from build123d import *

# Parameters (mm, degrees)
CROQUIS1_R              = 7.5
CROQUIS1_R_2            = 4.1
SALIENTE_EXTRUIR1_DEPTH = 24
CROQUIS2_W              = 0.35
CROQUIS2_H              = 1.1


with BuildPart() as part:
    # Croquis1 → Saliente-Extruir1 (new body)
    with BuildSketch(Plane(origin=(0, 0, 0), x_dir=(1, 0, 0), z_dir=(0, 1, 0))):
        with Locations(Location((0, 0, 0), (0, 0, 270))):
            Circle(CROQUIS1_R)
        with Locations(Location((0, 0, 0), (0, 0, 270))):
            Circle(CROQUIS1_R_2, mode=Mode.SUBTRACT)
    extrude(amount=SALIENTE_EXTRUIR1_DEPTH)

    # Croquis2 → Cortar-Revolución1 (revolve, cut)
    with BuildSketch(Plane.XY, mode=Mode.PRIVATE) as cortar_revoluci_n1_sk:
        with Locations((-7.325, 20.15)):
            Rectangle(CROQUIS2_W, CROQUIS2_H)
        with Locations((-7.325, 3.85)):
            Rectangle(CROQUIS2_W, CROQUIS2_H)
    revolve(cortar_revoluci_n1_sk.sketch.rotate(Axis((0, 0, 0), (0, 1, 0)), 270), axis=Axis((0, 0, 0), (0, 1, 0)), mode=Mode.SUBTRACT)


solid = part.part
Input: part model. Units: mm. Frame: model coordinates. A direction names the side the tool comes from. Round coordinates to 2 decimals unless told otherwise and drop trailing zeros. Loops run counter-clockwise (first coordinate to the right, second up) from the corner with the lowest first, then second, coordinate; pieces in that order, holes last. Notation, with made-up numbers: (-12, 39.25) -> (10, 39.25) arc R7 cw to (10, 50.25) -> close; hole circle Ø7 at (-27.75, -14.75). An arc over 180 degrees is marked (long way). Answer as a JSON object with one key per item and string values. Group by question number.
1) Draft query along Y for faces 1 (the flat face through (-3.2, 24, 3.2)), 2 (the cylindrical face through (-7.09, 20.16, 0.93)), 3 (the flat face through (-3.2, 0, 3.2)), 4 (the cylindrical face through (4.065, 11.832, -0.534)). Return one class per face: +Y half, -Y half, draft (parallel to the pull), parting line (faces both ways), or undercut.
2) Section query C-C on y = 16.75. Output: boundary loops of the cut face in (x, z).
3) Section query B-B on x = 0. Output: boundary loops of the cut face in (y, z), plus the area to 3 significant figures.
4) Section query D-D on x = -5.25. Output: boundary loops of the cut face in (y, z).
5) Reachability of faces 5 (the cylindrical face through (0.33, 22.327, -7.493)), 6 (the cylindrical face through (-7.09, 3.86, 0.93)) from +Z, -Z, +X, -X, +Y, -Y: full face, straight path, thin tool, end or side. Return the list, or none.
6) Ray query, L1, parallel to X at y = 9.25, z = 0; L2, parallel to Z at x = 2.5, y = 7; L3, parallel to Z at x = -3.5, y = 6. Return the intervals inside material, ascending.
7) Section query A-A on z = 0. Output: boundary loops of the cut face in (x, y).
8) Pin query (flat end, axial travel): pin 1 (6 mm diameter, centred on y = 5.5, z = 5.5, fed in from -X); pin 2 (1.5 mm diameter, centred on x = 2, y = 9.5, fed in from -Z); pin 3 (1 mm diameter, centred on y = 7.5, z = -4.5, fed in from +X). Return the tip coordinate at first contact, or that it passes through.
Reply:
{
 "1": {"face 1": "+Y half", "face 2": "undercut", "face 3": "-Y half", "face 4": "draft"},
 "2": {"outline": "circle Ø15 at (0, 0); hole circle Ø8.2 at (0, 0)"},
 "3": {"outline": "(0, -7.5) -> (3.3, -7.5) -> (3.3, -7.15) -> (4.4, -7.15) -> (4.4, -7.5) -> (19.6, -7.5) -> (19.6, -7.15) -> (20.7, -7.15) -> (20.7, -7.5) -> (24, -7.5) -> (24, -4.1) -> (0, -4.1) -> close; (0, 4.1) -> (24, 4.1) -> (24, 7.5) -> (20.7, 7.5) -> (20.7, 7.15) -> (19.6, 7.15) -> (19.6, 7.5) -> (4.4, 7.5) -> (4.4, 7.15) -> (3.3, 7.15) -> (3.3, 7.5) -> (0, 7.5) -> close", "area": "162 mm2"},
 "4": {"outline": "(0, -5.36) -> (3.3, -5.36) -> (3.3, -4.85) -> (4.4, -4.85) -> (4.4, -5.36) -> (19.6, -5.36) -> (19.6, -4.85) -> (20.7, -4.85) -> (20.7, -5.36) -> (24, -5.36) -> (24, 5.36) -> (20.7, 5.36) -> (20.7, 4.85) -> (19.6, 4.85) -> (19.6, 5.36) -> (4.4, 5.36) -> (4.4, 4.85) -> (3.3, 4.85) -> (3.3, 5.36) -> (0, 5.36) -> close"},
 "5": {"face 5": "+Y, -Y", "face 6": "none"},
 "6": {"L1": "x = -7.5 to -4.1, 4.1 to 7.5", "L2": "z = -7.07 to -3.25, 3.25 to 7.07", "L3": "z = -6.63 to -2.14, 2.14 to 6.63"},
 "7": {"outline": "(-7.5, 0) -> (-4.1, 0) -> (-4.1, 24) -> (-7.5, 24) -> (-7.5, 20.7) -> (-7.15, 20.7) -> (-7.15, 19.6) -> (-7.5, 19.6) -> (-7.5, 4.4) -> (-7.15, 4.4) -> (-7.15, 3.3) -> (-7.5, 3.3) -> close; (4.1, 0) -> (7.5, 0) -> (7.5, 3.3) -> (7.15, 3.3) -> (7.15, 4.4) -> (7.5, 4.4) -> (7.5, 19.6) -> (7.15, 19.6) -> (7.15, 20.7) -> (7.5, 20.7) -> (7.5, 24) -> (4.1, 24) -> close"},
 "8": {"pin 1": "stops at x = -7.07", "pin 2": "stops at z = -7.4", "pin 3": "stops at x = 6.34"}
}
